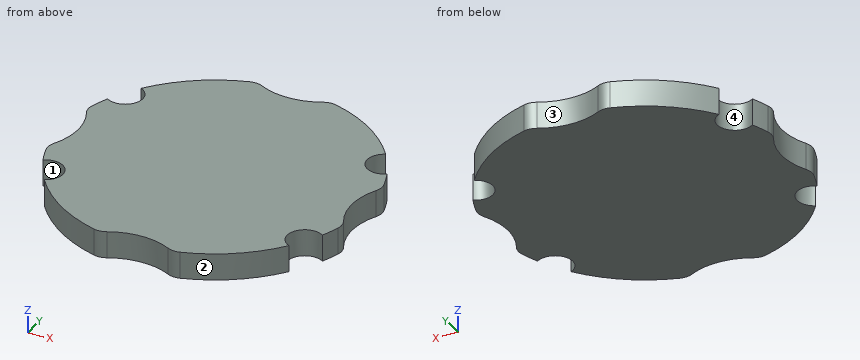
from build123d import *

# Parameters (mm, degrees)
BOSS_EXTRUDE1_DEPTH = 1.6
FILLET1_R           = 1
SKETCH2_R           = 1.05
CUT_EXTRUDE1_DEPTH  = 13.572804314


with BuildPart() as part:
    # Sketch1 → Boss-Extrude1 (new body)
    with BuildSketch(Plane.XY):
        with BuildLine():
            ThreePointArc((2.158317505, -8.891803279), (6.470027048, -6.470027048), (8.891803279, -2.158317505))
            ThreePointArc((8.891803279, -2.158317505), (8.25, 0), (8.891803279, 2.158317505))
            ThreePointArc((8.891803279, 2.158317505), (6.470027048, 6.470027048), (2.158317505, 8.891803279))
            ThreePointArc((2.158317505, 8.891803279), (0, 8.25), (-2.158317505, 8.891803279))
            ThreePointArc((-2.158317505, 8.891803279), (-6.470027048, 6.470027048), (-8.891803279, 2.158317505))
            ThreePointArc((-8.891803279, 2.158317505), (-8.25, 0), (-8.891803279, -2.158317505))
            ThreePointArc((-8.891803279, -2.158317505), (-6.470027048, -6.470027048), (-2.158317505, -8.891803279))
            ThreePointArc((-2.158317505, -8.891803279), (0, -8.25), (2.158317505, -8.891803279))
        make_face()
    extrude(amount=BOSS_EXTRUDE1_DEPTH)

    # Fillet1
    fillet1_edges = [part.edges().sort_by_distance(p)[0] for p in [
        (-2.158317505, -8.891803279, 0.8),
        (-8.891803279, -2.158317505, 0.8),
        (-8.891803279, 2.158317505, 0.8),
        (-2.158317505, 8.891803279, 0.8),
        (2.158317505, 8.891803279, 0.8),
        (8.891803279, 2.158317505, 0.8),
        (8.891803279, -2.158317505, 0.8),
        (2.158317505, -8.891803279, 0.8),
    ]]
    fillet(fillet1_edges, radius=FILLET1_R)

    # Sketch2 → Cut-Extrude1 (cut, through all)
    with BuildSketch(Plane.XY.offset(1.6)):
        with Locations((7.8, 4.5)):
            Circle(SKETCH2_R)
        with Locations((7.8, -4.5)):
            Circle(SKETCH2_R)
        with Locations((-7.8, -4.5)):
            Circle(SKETCH2_R)
        with Locations((-7.8, 4.5)):
            Circle(SKETCH2_R)
    extrude(amount=-CUT_EXTRUDE1_DEPTH, mode=Mode.SUBTRACT)


solid = part.part
CAD build for the part. Positions are in the model's coordinates, mm. Face numbers are marked on the shaded views. Give positions to 0.01 mm unless a question says otherwise; leave off trailing zeros. Order: outer loops, then holes, each group sorted by start corner. A loop starts at its lowest first (then second) coordinate and runs counter-clockwise, first axis right, second up. Notation, with made-up numbers: (-27, 35) -> (13, 35) arc R10 ccw to (13, 40) -> close; hole circle Ø4 at (15.5, 41.25). An arc over 180 degrees is marked (long way). Return JSON: item names as keys, results as strings.
Q1. Mould opens along Y. For the marked faces 1, 2, 3 and 4 say: pulls with the +Y half, pulls with the -Y half, needs draft (parallel to the pull), parting line crosses it, or undercut.
Working result:
{"face 1": "undercut", "face 2": "pulls with the -Y half", "face 3": "pulls with the +Y half", "face 4": "undercut"}
Q2. Drill centre lines: line 1 (Y direction, x = -7.8, z = 1.2); line 2 (X direction, y = -4.5, z = 0.6); line 3 (X direction, y = -1.25, z = 1.55). Where is each one in solid material? Low to high.
Working result:
{"line 1": "-3.45 to 3.45", "line 2": "-6.75 to 6.75", "line 3": "-8.45 to 8.45"}
Q3. Saw through at C-C (x = -7.8). Write the cut outline in (y, z), then the cut area to 3 significant figures.
Working result:
{"outline": "(-3.45, 0) -> (3.45, 0) -> (3.45, 1.6) -> (-3.45, 1.6) -> close", "area": "11.0 mm²"}
Q4. Flat gauge pin, fed straight in: pin 1 (1.9 mm diameter, centred on x = 7.8, y = 4.5, fed in from +Z). Where does the tip first touch, or does it go through?
Working result:
{"pin 1": "through"}
Q5. Saw through at B-B (y = -4.5). Write the cut outline in (x, z).
Working result:
{"outline": "(-6.75, 0) -> (6.75, 0) -> (6.75, 1.6) -> (-6.75, 1.6) -> close"}
Q6. Saw through at A-A (x = 7). Write the cut outline in (y, z).
Working result:
{"outline": "(-5.89, 0) -> (-5.18, 0) -> (-5.18, 1.6) -> (-5.89, 1.6) -> close; (-3.82, 0) -> (3.82, 0) -> (3.82, 1.6) -> (-3.82, 1.6) -> close; (5.18, 0) -> (5.89, 0) -> (5.89, 1.6) -> (5.18, 1.6) -> close"}
